Autodesk Inventor part; units mm, degrees
ref_plane "YZ Plane" through (0, 0, 0) normal (1, 0, 0) x (0, 1, 0)
ref_plane "XZ Plane" through (0, 0, 0) normal (0, 1, 0) x (-1, 0, 0)
ref_plane "XY Plane" through (0, 0, 0) normal (0, 0, 1) x (1, 0, 0)
sketch "Esboço1" plane through (0, 0, 0) normal (0, 0, 1) x (1, 0, 0)
  line L0 (-2, 7.5) -> (2, 7.5)
  line L1 (2, 7.5) -> (2, -7.5)
  line L2 (2, -7.5) -> (-2, -7.5)
  line L3 (-2, -7.5) -> (-2, 7.5)
  line L4 (-2, 7.5) -> (2, -7.5) construction
  line L5 (2, 7.5) -> (-2, -7.5) construction
  point P0 (0, 0)
  dimension "d0" = 4
  dimension "d1" = 15
extrude "Extrusão1" add sketch "Esboço1" along normal blind 1
sketch "Esboço2" plane through (0, 0, 1) normal (0, 0, 1) x (1, 0, 0)
  line L0 (-1.95, 6.95) -> (1.95, 6.95)
  line L1 (1.95, 6.95) -> (1.95, -6.95)
  line L2 (1.95, -6.95) -> (-1.95, -6.95)
  line L3 (-1.95, -6.95) -> (-1.95, 6.95)
  line L4 (-1.95, 6.95) -> (1.95, -6.95) construction
  line L5 (1.95, 6.95) -> (-1.95, -6.95) construction
  point P0 (0, 0)
  dimension "d4" = 3.9
  dimension "d5" = 13.9
extrude "Extrusão2" add sketch "Esboço2" along normal blind 5
sketch "Esboço3" plane through (0, 0, 6) normal (0, 0, 1) x (1, 0, 0)
  circle A0 centre (0, 0) radius 1.95
  line L0 (1.95, -6.95) -> (-1.95, -6.95)
  line L1 (-0.5, 6.95) -> (0.5, 6.95)
  line L2 (0.5, 6.95) -> (0.5, -6.95)
  line L3 (0.5, -6.95) -> (-0.5, -6.95)
  line L4 (-0.5, -6.95) -> (-0.5, 6.95)
  line L5 (-0.5, 6.95) -> (0.5, -6.95) construction
  line L6 (0.5, 6.95) -> (-0.5, -6.95) construction
  line L7 (-1.95, 6.95) -> (1.95, 6.95)
  line L8 (1.95, 6.95) -> (1.95, -6.95)
  line L9 (1.95, -6.95) -> (-1.95, -6.95)
  line L10 (-1.95, -6.95) -> (-1.95, 6.95)
  line L11 (-1.95, 6.95) -> (1.95, -6.95) construction
  line L12 (1.95, 6.95) -> (-1.95, -6.95) construction
  point P0 (-1.95, 0)
  point P1 (-0.5, -1.8848)
  point P2 (-0.5, 1.8848)
  point P3 (1.95, 0)
  point P4 (0.5, 1.8848)
  point P5 (0.5, -1.8848)
  dimension "d8" = 3.9
  dimension "d9" = 1
extrude "Extrusão3" cut sketch "Esboço3" against normal blind 5 contours L8 L0 L2 A0 | A0 L2 L7 L8 | A0 L10 L7 L4 | L4 L0 L10 A0
sketch "Esboço4" plane through (0, 0, 6) normal (0, 0, 1) x (1, 0, 0)
  line L0 (-0.5, -4.5) -> (0.5, -4.5)
  line L1 (0.5, -4.5) -> (0.5, 4.5)
  line L2 (0.5, 4.5) -> (-0.5, 4.5)
  line L3 (-0.5, 4.5) -> (-0.5, -4.5)
  line L4 (-0.5, -4.5) -> (0.5, 4.5) construction
  line L5 (0.5, -4.5) -> (-0.5, 4.5) construction
  line L6 (0.5, 1.8848) -> (0.5, 6.95)
  line L7 (-0.5, -6.95) -> (0.5, -6.95)
  line L8 (0.5, -6.95) -> (0.5, 6.95)
  line L9 (0.5, 6.95) -> (-0.5, 6.95)
  line L10 (-0.5, 6.95) -> (-0.5, -6.95)
  line L11 (-0.5, -6.95) -> (0.5, 6.95) construction
  line L12 (0.5, -6.95) -> (-0.5, 6.95) construction
  point P0 (0, 0)
  dimension "d12" = 1
  dimension "d13" = 9
extrude "Extrusão4" cut sketch "Esboço4" against normal blind 3 contours L0 L8 L7 L10 | L10 L9 L6 L2
sketch "Esboço5" plane through (0, 0, 0) normal (0, 0, -1) x (-1, 0, 0)
  point P0 (0, 0)
  point P1 (0, 0)
  dimension "d23" = 0
  dimension "d24" = 0
hole "Furo1" at (0, 0, 0) direction (0, 0, 1) diameter 2.459 end through all
properties part number "TRAVA"
Source: CAD feature listing. Evaluate the final solid. Frame: model axes, mm. A direction names the side the tool comes from. Give positions to 0.01 mm unless a question says otherwise; leave off trailing zeros. Write each loop counter-clockwise with the first axis right and the second up, starting at its lowest first coordinate (ties: lowest second). Pieces come first, ordered by that corner, then holes. Notation, with made-up numbers: (-21, -31.75) -> (-5, -31.75) arc R32 ccw to (-5, 5.25) -> close; hole circle Ø6 at (87.5, -13). An arc over 180 degrees is marked (long way). Return JSON: item names as keys, results as strings. Group by question number.
1. Section B-B, the plane y = 0. Output: boundary loops of the cut face in (x, z), then the cut area to 3 significant figures.
2. Material intervals for line 1 (Y direction, x = -0.1, z = 4.5); line 2 (Y direction, x = 0, z = 2.25); line 3 (X direction, y = -5.25, z = 2), sorted ascending. Write a range as from..to.
3. Section D-D, the plane y = -4.25. Output: boundary loops of the cut face in (x, z), then the cut area to 3 significant figures.
4. Pin query (flat end, axial travel): pin 1 Ø0.8 at (x, z) = (0, 2) entering from +Y; pin 2 Ø2.5 at (y, z) = (3.5, 3.5) entering from +X; pin 3 Ø0.5 at (x, z) = (0, 2.5) entering from -Y. Return the tip coordinate at first contact, or that it passes through.
5. Mould query, pull axis Y, two halves, no side actions, for faces 6 (the face through (-0.5, -4, 3)), 7 (the face through (0, 4.5, 5)), 8 (the face through (0, -4.5, 5)), 9 (the face through (0.748, -0.976, 3.042)). Classes: +Y half, -Y half, draft (parallel to the pull), parting line (faces both ways), or undercut.
6. Access query for faces 1 (the face through (0.5, 4, 3)), 2 (the face through (-1.95, 0.04, 3.54)), 3 (the face through (0, 6, 3)), 4 (the face through (-0.5, 4, 3)), 5 (the face through (0, -6, 3)). Directions: +Z, -Z, +X, -X, +Y, -Y. A direction counts if a zero-diameter tool reaches every point of the face in a straight line with its end or side. Return the directions, or none.
7. Section C-C, the plane z = 2.4. Output: boundary loops of the cut face in (x, y).
8. Section A-A, the plane x = 0. Output: boundary loops of the cut face in (y, z).
Determined:
{
 "1": {"outline": "(-2, 0) -> (-1.23, 0) -> (-1.23, 6) -> (-1.95, 6) -> (-1.95, 1) -> (-2, 1) -> close; (1.23, 0) -> (2, 0) -> (2, 1) -> (1.95, 1) -> (1.95, 6) -> (1.23, 6) -> close", "area": "8.75 mm2"},
 "2": {"line 1": "y = -4.5..-1.23, 1.23..4.5", "line 2": "y = -6.95..-1.23, 1.23..6.95", "line 3": "x = -0.5..0.5"},
 "3": {"outline": "(-2, 0) -> (2, 0) -> (2, 1) -> (0.5, 1) -> (0.5, 6) -> (-0.5, 6) -> (-0.5, 1) -> (-2, 1) -> close", "area": "9.00 mm2"},
 "4": {"pin 1": "stops at y = 6.95", "pin 2": "stops at x = 0.5", "pin 3": "stops at y = -6.95"},
 "5": {"face 6": "draft", "face 7": "+Y half", "face 8": "-Y half", "face 9": "undercut"},
 "6": {"face 1": "+Z, +X, +Y", "face 2": "+Z, -X", "face 3": "+Z, +X, -X, +Y", "face 4": "+Z, -X, +Y", "face 5": "+Z, +X, -X, -Y"},
 "7": {"outline": "(-0.5, -6.95) -> (0.5, -6.95) -> (0.5, -1.88) arc R1.95 ccw to (0.5, 1.88) -> (0.5, 6.95) -> (-0.5, 6.95) -> (-0.5, 1.88) arc R1.95 ccw to (-0.5, -1.88) -> close; hole circle Ø2.46 at (0, 0)"},
 "8": {"outline": "(-7.5, 0) -> (-1.23, 0) -> (-1.23, 6) -> (-4.5, 6) -> (-4.5, 3) -> (-6.95, 3) -> (-6.95, 1) -> (-7.5, 1) -> close; (1.23, 0) -> (7.5, 0) -> (7.5, 1) -> (6.95, 1) -> (6.95, 3) -> (4.5, 3) -> (4.5, 6) -> (1.23, 6) -> close"}
}
